Check sheet for the drawn part. Datum: minimum x, y, z corner. Units: mm. A direction names the side the tool comes from. Coordinates: 2 decimals unless noted, no trailing zeros. Order: outer loops, then holes, each group sorted by start corner. A loop starts at its lowest first (then second) coordinate and runs counter-clockwise, first axis right, second up. Notation, with made-up numbers: (22, 38) - (76, 38) arc R18 cw to (76, 51) - close; hole circle Ø9 at (-16, -23). An arc over 180 degrees is marked (long way). Answer as CSV lines item,"result". Start each with the question number.
1. Set-up check for the marked faces 1 and 2: record each of +Z, -Z, +X, -X, +Y, -Y from which the full face is reachable in a straight line by a thin tool's end or side.
2. Section check C-C (x = 14). Record the cut outline in (y, z).
3. Mould release check, pull along X, two halves, no side actions. Record for the marked faces 3, 4 and 5: pulls with the +X half, pulls with the -X half, needs draft (parallel to the pull), parting line crosses it, or undercut.
4. Section check D-D (z = 23.25). Record the cut outline in (x, y).
5. Section check B-B (y = 0.7). Record the cut outline in (x, z).
6. Material ranges on L1, parallel to X at y = 1.3, z = 14; L2, parallel to X at y = 0.3, z = 24.5; L3, parallel to X at y = 1.25, z = 15, recorded low to high. Write a range as [from, to].
7. Go/stop test with flat-tipped pins: pin 1 (0.6 mm diameter, centred on y = 1, z = 7, fed in from +X); pin 2 (0.6 mm diameter, centred on x = 22.5, y = 0.5, fed in from +Z); pin 3 (2 mm diameter, centred on x = 24.5, z = 18, fed in from -Y); pin 4 (1 mm diameter, centred on y = 1, z = 3, fed in from +X). Record where each tip stops, or that it passes through.
8. Section check A-A (z = 14). Record the cut outline in (x, y), and give its area (3 significant figures).
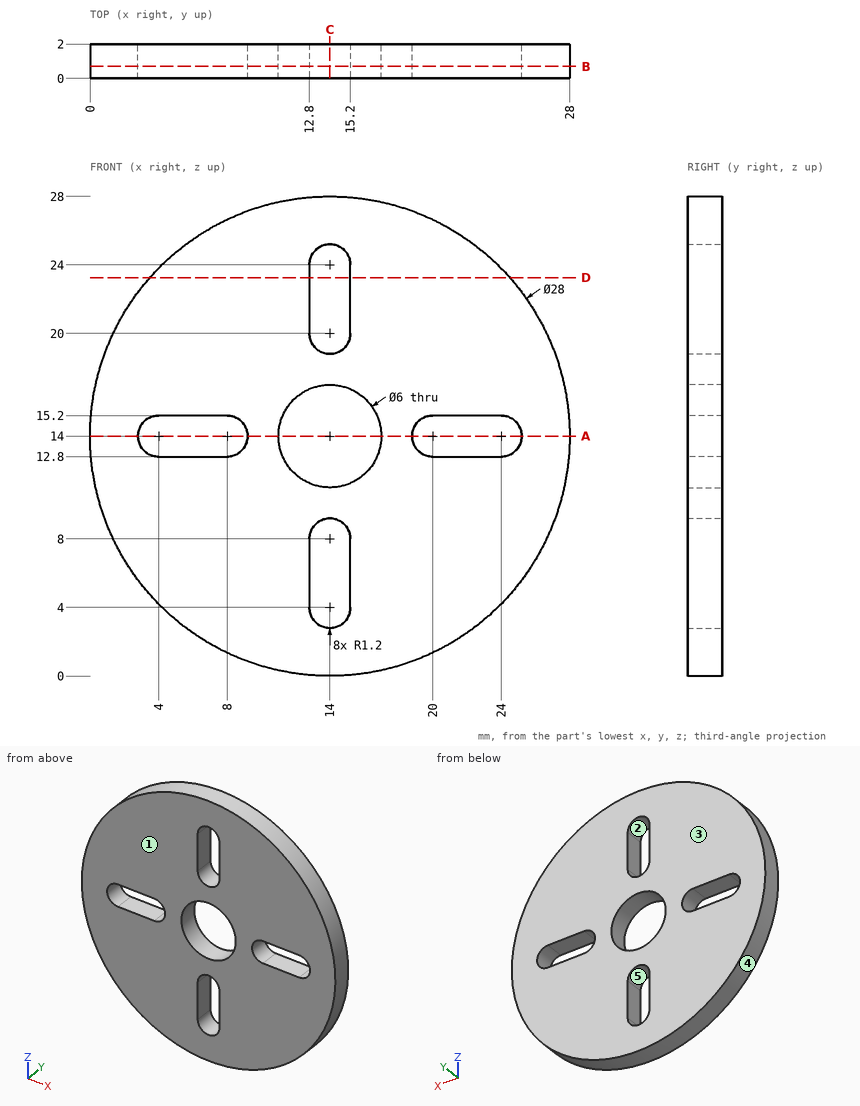
Evaluation:
1,face 1,"+Z, -Z, +X, -X, -Y"
1,face 2,"+Y, -Y"
2,outline,"(0, 0) - (2, 0) - (2, 2.8) - (0, 2.8) - close; (0, 9.2) - (2, 9.2) - (2, 11) - (0, 11) - close; (0, 17) - (2, 17) - (2, 18.8) - (0, 18.8) - close; (0, 25.2) - (2, 25.2) - (2, 28) - (0, 28) - close"
3,face 3,"needs draft"
3,face 4,"parting line crosses it"
3,face 5,"undercut"
4,outline,"(3.49, 0) - (12.8, 0) - (12.8, 2) - (3.49, 2) - close; (15.2, 0) - (24.51, 0) - (24.51, 2) - (15.2, 2) - close"
5,outline,"circle Ø28 at (14, 14); hole (4, 12.8) - (8, 12.8) arc R1.2 ccw to (8, 15.2) - (4, 15.2) arc R1.2 ccw to start; hole circle Ø6 at (14, 14); hole (12.8, 4) arc R1.2 ccw to (15.2, 4) - (15.2, 8) arc R1.2 ccw to (12.8, 8) - close; hole (12.8, 20) arc R1.2 ccw to (15.2, 20) - (15.2, 24) arc R1.2 ccw to (12.8, 24) - close; hole (20, 12.8) - (24, 12.8) arc R1.2 ccw to (24, 15.2) - (20, 15.2) arc R1.2 ccw to start"
6,L1,"x = [0, 2.8], [9.2, 11], [17, 18.8], [25.2, 28]"
6,L2,"x = [4.74, 12.91], [15.09, 23.26]"
6,L3,"x = [0.04, 3.34], [8.66, 11.17], [16.83, 19.34], [24.66, 27.96]"
7,pin 1,"stops at x = 26.29"
7,pin 2,"stops at z = 25.35"
7,pin 3,"stops at y = 0"
7,pin 4,"stops at x = 23.26"
8,outline,"(0, 0) - (2.8, 0) - (2.8, 2) - (0, 2) - close; (9.2, 0) - (11, 0) - (11, 2) - (9.2, 2) - close; (17, 0) - (18.8, 0) - (18.8, 2) - (17, 2) - close; (25.2, 0) - (28, 0) - (28, 2) - (25.2, 2) - close"
8,area,"18.4 mm²"
